Verification items for the finished model (mm, model axes). Face numbers are marked on the shaded views. A direction names the side the tool comes from. Coordinates: 2 decimals unless noted, no trailing zeros. Write each loop counter-clockwise with the first axis right and the second up, starting at its lowest first coordinate (ties: lowest second). Pieces come first, ordered by that corner, then holes. Notation, with made-up numbers: (-15.75, 8) -> (35.25, 8) arc R19 ccw to (35.25, 43) -> close; hole circle Ø8 at (13, 64.25). An arc over 180 degrees is marked (long way). Use CSV: the item, a comma, the result in double quotes.
```python
from build123d import *

# Parameters (mm, degrees)
BOSS_EXTRU_1_DEPTH      = 10
ENL_V_MAT_EXTRU_2_DEPTH = 3
ESQUISSE5_R             = 2.05
ENL_V_MAT_EXTRU_3_DEPTH = 12.82423359


with BuildPart() as part:
    # Esquisse1 → Boss.-Extru.1 (new body)
    with BuildSketch(Plane(origin=(0, 0, 0), x_dir=(1, 0, 0), z_dir=(0, 1, 0))):
        Polygon((3.75, 0), (-3.75, 0), (-5.25, 1.5), (-5.25, 3.5), (5.25, 3.5), (5.25, 1.5), align=None)
    extrude(amount=BOSS_EXTRU_1_DEPTH)

    # Esquisse4 → Enlèv. mat.-Extru.2 (cut)
    with BuildSketch(Plane.XY):
        Polygon((3.55, 7.049593456), (0, 9.099186911), (-3.55, 7.049593456), (-3.55, 2.950406544), (0, 0.900813089), (3.55, 2.950406544), align=None)
    extrude(amount=-ENL_V_MAT_EXTRU_2_DEPTH, mode=Mode.SUBTRACT)

    # Esquisse5 → Enlèv. mat.-Extru.3 (cut, through all)
    with BuildSketch(Plane(origin=(0, 0, -3.5), x_dir=(-1, 0, 0), z_dir=(0, 0, -1))):
        with Locations((0, 5)):
            Circle(ESQUISSE5_R)
    extrude(amount=-ENL_V_MAT_EXTRU_3_DEPTH, mode=Mode.SUBTRACT)


solid = part.part
```
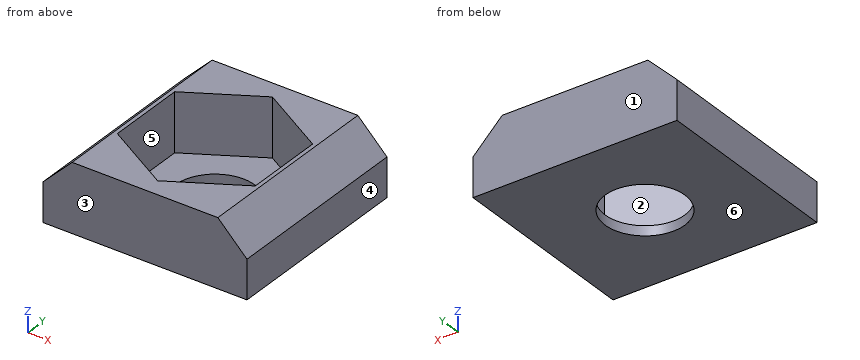
1) Cross-section at A-A (z = -2.2). Record the boundary of the cut face in (x, y), plus the area to 3 significant figures.
Return value:
outline,"(-5.25, 0) -> (5.25, 0) -> (5.25, 10) -> (-5.25, 10) -> close; hole (-3.55, 2.95) -> (0, 0.9) -> (3.55, 2.95) -> (3.55, 7.05) -> (0, 9.1) -> (-3.55, 7.05) -> close"
area,"61.3 mm2"
2) Mould release check, pull along Y, two halves, no side actions. Record for the marked faces 1, 2, 3 and 4: released by +Y, released by -Y, zero draft, split by the parting line, or undercut.
Return value:
face 1,"released by +Y"
face 2,"undercut"
face 3,"released by -Y"
face 4,"zero draft"
3) Set-up check for the marked faces 5 and 6: record each of +Z, -Z, +X, -X, +Y, -Y from which the full face is reachable in a straight line by a thin tool's end or side.
Return value:
face 5,"+Z"
face 6,"-Z, +X, -X, +Y, -Y"
4) Gauge pin test, flat end, axial feed: pin 1 (2 mm diameter, centred on x = -1.5, y = 4, fed in from +Z). Record the tip position at first contact, or that the pin passes through.
Return value:
pin 1,"z = -3"
5) Cross-section at C-C (x = 1). Record the boundary of the cut face in (y, z), plus the area to 3 significant figures.
Return value:
outline,"(0, -3.5) -> (3.21, -3.5) -> (3.21, -3) -> (1.48, -3) -> (1.48, 0) -> (0, 0) -> close; (6.79, -3.5) -> (10, -3.5) -> (10, 0) -> (8.52, 0) -> (8.52, -3) -> (6.79, -3) -> close"
area,"12.1 mm2"
6) Scan lines: L1, parallel to X at y = 4.5, z = -2.3; L2, parallel to Y at x = 0, z = -3.05; L3, parallel to Y at x = -3, z = -1.7. Record each from-to range of solid material in increasing order.
Return value:
L1,"-5.25 to -3.55, 3.55 to 5.25"
L2,"0 to 2.95, 7.05 to 10"
L3,"0 to 2.63, 7.37 to 10"
7) Cross-section at D-D (z = -1). Record the boundary of the cut face in (x, y), plus the area to 3 significant figures.
Return value:
outline,"(-4.75, 0) -> (4.75, 0) -> (4.75, 10) -> (-4.75, 10) -> close; hole (-3.55, 2.95) -> (0, 0.9) -> (3.55, 2.95) -> (3.55, 7.05) -> (0, 9.1) -> (-3.55, 7.05) -> close"
area,"51.3 mm2"
8) Cross-section at B-B (y = 4.5). Record the boundary of the cut face in (x, z), plus the area to 3 significant figures.
Return value:
outline,"(-5.25, -3.5) -> (-1.99, -3.5) -> (-1.99, -3) -> (-3.55, -3) -> (-3.55, 0) -> (-3.75, 0) -> (-5.25, -1.5) -> close; (1.99, -3.5) -> (5.25, -3.5) -> (5.25, -1.5) -> (3.75, 0) -> (3.55, 0) -> (3.55, -3) -> (1.99, -3) -> close"
area,"11.2 mm2"
